Source: CAD feature listing. Evaluate the final solid. Frame: model axes, mm. Face numbers are marked on the shaded views. A direction names the side the tool comes from. Give positions to 0.01 mm unless a question says otherwise; leave off trailing zeros. Order: outer loops, then holes, each group sorted by start corner. A loop starts at its lowest first (then second) coordinate and runs counter-clockwise, first axis right, second up.
Autodesk Inventor part; units mm, degrees
ref_plane "YZ Plane" through (0, 0, 0) normal (1, 0, 0) x (0, 1, 0)
ref_plane "XZ Plane" through (0, 0, 0) normal (0, 1, 0) x (-1, 0, 0)
ref_plane "XY Plane" through (0, 0, 0) normal (0, 0, 1) x (1, 0, 0)
sketch "Sketch1" plane through (0, 0, 0) normal (0, 1, 0) x (-1, 0, 0)
  line L0 (-20.5, 52.5) -> (20.5, 52.5)
  line L1 (20.5, 52.5) -> (20.5, -52.5)
  line L2 (20.5, -52.5) -> (-20.5, -52.5)
  line L3 (-20.5, -52.5) -> (-20.5, 52.5)
  line L4 (-20.5, 52.5) -> (20.5, -52.5) construction
  line L5 (20.5, 52.5) -> (-20.5, -52.5) construction
  line L6 (-23.5, 55.5) -> (23.5, 55.5)
  line L7 (23.5, 55.5) -> (23.5, -55.5)
  line L8 (23.5, -55.5) -> (-23.5, -55.5)
  line L9 (-23.5, -55.5) -> (-23.5, 55.5)
  line L10 (-23.5, 55.5) -> (23.5, -55.5) construction
  line L11 (23.5, 55.5) -> (-23.5, -55.5) construction
  point P0 (0, 0)
  dimension "d0" = 41
  dimension "d1" = 105
  dimension "d4" = 47
  dimension "d5" = 111
extrude "Extrusion1" add sketch "Sketch1" along normal blind 3 contours L0 L1 L2 L3
sketch "Sketch3" plane through (0, 3, 0) normal (0, 1, 0) x (1, 0, 0)
  line L0 (23.5, -55.5) -> (-23.5, -55.5)
  line L1 (-23.5, -55.5) -> (-23.5, 55.5)
  line L2 (-23.5, 55.5) -> (23.5, 55.5)
  line L3 (23.5, 55.5) -> (23.5, -55.5)
  line L4 (23.5, -55.5) -> (-23.5, 55.5) construction
  line L5 (-23.5, -55.5) -> (23.5, 55.5) construction
  line L6 (20.5, 52.5) -> (-20.5, 52.5)
  line L7 (20.5, -52.5) -> (-20.5, -52.5)
  line L8 (-20.5, -52.5) -> (-20.5, 52.5)
  line L9 (-20.5, 52.5) -> (20.5, 52.5)
  line L10 (20.5, 52.5) -> (20.5, -52.5)
  line L11 (20.5, -52.5) -> (-20.5, 52.5) construction
  line L12 (-20.5, -52.5) -> (20.5, 52.5) construction
  point P0 (0, 0)
  dimension "d6" = 47
  dimension "d7" = 111
extrude "Extrusion3" add sketch "Sketch3" against normal blind 65
sketch "Sketch4" plane through (23.5, 3, -55.5) normal (0, 0, -1) x (-1, 0, 0)
  line L0 (0, 0) -> (23.5, 0) construction
  line L1 (23.5, 0) -> (23.5, -48) construction
  line L2 (23.5, -48) -> (14.75, -48) construction
  line L3 (23.5, -48) -> (32.25, -48) construction
  circle A0 centre (14.75, -48) radius 2
  circle A1 centre (32.25, -48) radius 2
  point P0 (23.5, -3)
  dimension "d12" = 23.5
  dimension "d13" = 48
  dimension "d14" = 8.75
  dimension "d15" = 8.75
  dimension "d16" = 4
  dimension "d17" = 4
extrude "Extrusion4" cut sketch "Sketch4" against normal blind 3
sketch "Sketch5" plane through (-23.5, 3, 55.5) normal (0, 0, 1) x (1, 0, 0)
  line L0 (47, 0) -> (47, -65) construction
  line L1 (47, 0) -> (23.5, 0) construction
  line L2 (0, 0) -> (47, 0) construction
  line L3 (23.5, 0) -> (23.5, -48) construction
  line L4 (23.5, 0) -> (71.5, 0) construction
  circle A0 centre (32.25, -48) radius 2
  line L5 (23.5, -48) -> (32.25, -48) construction
  circle A1 centre (14.75, -48) radius 2
  line L6 (23.5, -48) -> (14.75, -48) construction
  circle A2 centre (32.25, -48) radius 2 construction
  circle A3 centre (14.75, -48) radius 2 construction
  point P0 (23.5, -3)
  dimension "d20" = 23.5
  dimension "d21" = 48
  dimension "d22" = 90
extrude "Extrusion5" cut sketch "Sketch5" against normal blind 3
sketch "Sketch6" plane through (23.5, 3, 55.5) normal (1, 0, 0) x (0, 0, -1)
  line L0 (111, 0) -> (111, -65) construction
  line L1 (111, 0) -> (55.5, 0) construction
  line L2 (111, 0) -> (0, 0) construction
  line L3 (55.5, 0) -> (51.5, 0) construction
  line L4 (51.5, 0) -> (59.5, 0)
  line L5 (59.5, 0) -> (59.5, -8)
  line L6 (59.5, -8) -> (51.5, -8)
  line L7 (51.5, -8) -> (51.5, 0)
  line L8 (51.5, 0) -> (47.5, 0)
  line L9 (47.5, 0) -> (45.5, 0)
  line L10 (45.5, 0) -> (45.5, -8)
  line L11 (45.5, -8) -> (47.5, -8)
  line L12 (47.5, -8) -> (47.5, 0)
  line L13 (59.5, 0) -> (63.5, 0)
  line L14 (63.5, 0) -> (65.5, 0)
  line L15 (65.5, 0) -> (65.5, -8)
  line L16 (65.5, -8) -> (63.5, -8)
  line L17 (63.5, -8) -> (63.5, 0)
  point P0 (55.5, -3)
  dimension "d25" = 55.5
  dimension "d26" = 4
  dimension "d27" = 8
  dimension "d28" = 8
  dimension "d29" = 4
  dimension "d30" = 2
  dimension "d31" = 4
  dimension "d32" = 2
  dimension "d33" = 8
extrude "Extrusion6" cut sketch "Sketch6" against normal blind 3
sketch "Sketch7" plane through (20.5, 3, 55.5) normal (1, 0, 0) x (0, 0, -1)
  point P0 (55.5, -3)
sketch "Sketch8" plane through (20.5, 3, 55.5) normal (1, 0, 0) x (0, 0, -1)
  line L0 (65.5, 0) -> (65.5, -3)
  line L1 (63.5, -3) -> (59.5, -3)
  line L2 (65.5, 0) -> (63.5, 0)
  line L3 (63.5, 0) -> (63.5, -3)
  line L4 (63.5, -3) -> (65.5, -3)
  line L5 (65.5, -3) -> (65.5, 0)
  line L6 (51.5, 0) -> (59.5, 0)
  line L7 (51.5, -3) -> (51.5, 0)
  line L8 (59.5, 0) -> (51.5, 0)
  line L9 (51.5, 0) -> (51.5, -3)
  line L10 (51.5, -3) -> (59.5, -3)
  line L11 (59.5, -3) -> (59.5, 0)
  line L12 (51.5, 0) -> (47.5, 0)
  line L13 (45.5, -8) -> (45.5, 0)
  line L14 (47.5, 0) -> (45.5, 0)
  line L15 (45.5, 0) -> (45.5, -3)
  line L16 (45.5, -3) -> (47.5, -3)
  line L17 (47.5, -3) -> (47.5, 0)
  point P0 (55.5, -3)
extrude "Extrusion7" add sketch "Sketch8" along normal blind 3
sketch "Sketch9" plane through (23.5, 3, 55.5) normal (1, 0, 0) x (0, 0, -1)
  line L0 (59.5, -8) -> (51.5, -8)
  circle A0 centre (55.5, -8) radius 4
  point P0 (55.5, -3)
  dimension "d38" = 8
extrude "Extrusion8" cut sketch "Sketch9" against normal blind 3
sketch "Sketch10" plane through (0, 3, 0) normal (0, 1, 0) x (1, 0, 0)
  line L0 (-23.5, 55.5) -> (23.5, 55.5)
  line L1 (0, 55.5) -> (0, 40.5) construction
  line L2 (0, 40.5) -> (0, 35.5) construction
  line L3 (0, 35.5) -> (0, 30.5) construction
  line L4 (0, 30.5) -> (0, 25.5) construction
  line L5 (0, 25.5) -> (0, 20.5) construction
  line L6 (0, 20.5) -> (0, 15.5) construction
  line L7 (0, 15.5) -> (0, 10.5) construction
  line L8 (0, 10.5) -> (0, 5.5) construction
  line L9 (0, 5.5) -> (0, 0.5) construction
  line L10 (-15, 1.5) -> (15, 1.5)
  line L11 (15, 1.5) -> (15, -1.5)
  line L12 (15, -1.5) -> (-15, -1.5)
  line L13 (-15, -1.5) -> (-15, 1.5)
  line L14 (-15, 1.5) -> (15, -1.5) construction
  line L15 (15, 1.5) -> (-15, -1.5) construction
  line L16 (-15, 7) -> (15, 7)
  line L17 (15, 7) -> (15, 4)
  line L18 (15, 4) -> (-15, 4)
  line L19 (-15, 4) -> (-15, 7)
  line L20 (-15, 7) -> (15, 4) construction
  line L21 (15, 7) -> (-15, 4) construction
  line L22 (-15, 12) -> (15, 12)
  line L23 (15, 12) -> (15, 9)
  line L24 (15, 9) -> (-15, 9)
  line L25 (-15, 9) -> (-15, 12)
  line L26 (-15, 12) -> (15, 9) construction
  line L27 (15, 12) -> (-15, 9) construction
  line L28 (-15, 17) -> (15, 17)
  line L29 (15, 17) -> (15, 14)
  line L30 (15, 14) -> (-15, 14)
  line L31 (-15, 14) -> (-15, 17)
  line L32 (-15, 17) -> (15, 14) construction
  line L33 (15, 17) -> (-15, 14) construction
  line L34 (-15, 22) -> (15, 22)
  line L35 (15, 22) -> (15, 19)
  line L36 (15, 19) -> (-15, 19)
  line L37 (-15, 19) -> (-15, 22)
  line L38 (-15, 22) -> (15, 19) construction
  line L39 (15, 22) -> (-15, 19) construction
  line L40 (-15, 27) -> (15, 27)
  line L41 (15, 27) -> (15, 24)
  line L42 (15, 24) -> (-15, 24)
  line L43 (-15, 24) -> (-15, 27)
  line L44 (-15, 27) -> (15, 24) construction
  line L45 (15, 27) -> (-15, 24) construction
  line L46 (-15, 32) -> (15, 32)
  line L47 (15, 32) -> (15, 29)
  line L48 (15, 29) -> (-15, 29)
  line L49 (-15, 29) -> (-15, 32)
  line L50 (-15, 32) -> (15, 29) construction
  line L51 (15, 32) -> (-15, 29) construction
  line L52 (-15, 37) -> (15, 37)
  line L53 (15, 37) -> (15, 34)
  line L54 (15, 34) -> (-15, 34)
  line L55 (-15, 34) -> (-15, 37)
  line L56 (-15, 37) -> (15, 34) construction
  line L57 (15, 37) -> (-15, 34) construction
  line L58 (-15, 42) -> (15, 42)
  line L59 (15, 42) -> (15, 39)
  line L60 (15, 39) -> (-15, 39)
  line L61 (-15, 39) -> (-15, 42)
  line L62 (-15, 42) -> (15, 39) construction
  line L63 (15, 42) -> (-15, 39) construction
  point P0 (0, 0)
  dimension "d41" = 15
  dimension "d42" = 5
  dimension "d43" = 5
  dimension "d44" = 5
  dimension "d45" = 5
  dimension "d46" = 5
  dimension "d47" = 5
  dimension "d48" = 5
  dimension "d49" = 5
  dimension "d50" = 30
  dimension "d51" = 3
  dimension "d52" = 30
  dimension "d53" = 3
  dimension "d54" = 30
  dimension "d55" = 3
  dimension "d56" = 30
  dimension "d57" = 3
  dimension "d58" = 30
  dimension "d59" = 3
  dimension "d60" = 30
  dimension "d61" = 3
  dimension "d62" = 30
  dimension "d63" = 3
  dimension "d64" = 30
  dimension "d65" = 3
  dimension "d66" = 30
  dimension "d67" = 3
extrude "Extrusion9" cut sketch "Sketch10" against normal blind 3
properties part number "netzteil_case"
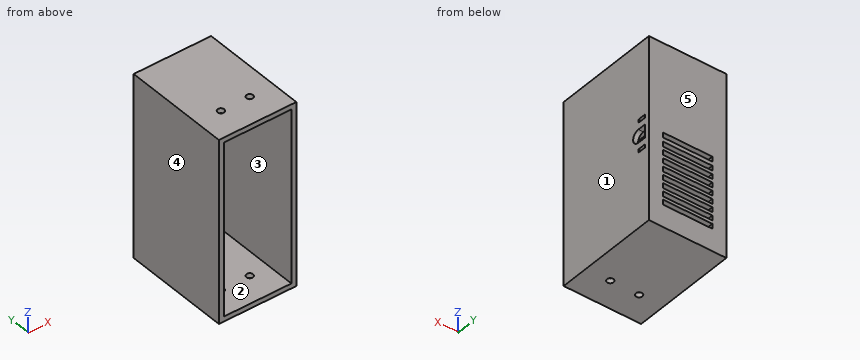
(1) Section A-A, the plane y = -45. Return loops of the section in (x, z), plus the area to 3 significant figures.
(2) Pin query (flat end, axial travel): pin 1 Ø4 at (x, z) = (15, 38) entering from -Y. Return the tip coordinate at first contact, or that it passes through.
(3) Section D-D, the plane x = 0. Count the separate pieces of the cut face and the enclosed holes in it, plus the area to 3 significant figures.
(4) Draft query along X for the marked faces 3, 4 and 5. Return one class per face: +X half, -X half, draft (parallel to the pull), parting line (faces both ways), or undercut.
(5) Section C-C, the plane y = -57. Return loops of the section in (x, z), plus the area to 3 significant figures.
(6) Section B-B, the plane z = 42. Return loops of the section in (x, y).
(7) Access query for the marked faces 1 and 2. Directions: +Z, -Z, +X, -X, +Y, -Y. A direction counts if a zero-diameter tool reaches every point of the face in a straight line with its end or side. Return the directions, or none.
(8) Line query: line 1 along Z through (x, y) = (9.5, -52.5); line 2 along X through (y, z) = (-52, 37.5); line 3 along Y through (x, z) = (-8.75, -53.6). Output: solid intervals per line, ascending.
Checks:
1. outline: (-23.5, -55.5) - (-10.75, -55.5) - (-10.75, -52.5) - (-20.5, -52.5) - (-20.5, 52.5) - (-10.75, 52.5) - (-10.75, 55.5) - (-23.5, 55.5) - close; (-6.75, -55.5) - (6.75, -55.5) - (6.75, -52.5) - (-6.75, -52.5) - close; (-6.75, 52.5) - (6.75, 52.5) - (6.75, 55.5) - (-6.75, 55.5) - close; (10.75, -55.5) - (23.5, -55.5) - (23.5, 55.5) - (10.75, 55.5) - (10.75, 52.5) - (20.5, 52.5) - (20.5, -52.5) - (10.75, -52.5) - close
1. area: 864 mm2
2. pin 1: stops at y = 0
3. separate pieces: 10
3. enclosed holes: 0
3. area: 624 mm2
4. face 3: undercut
4. face 4: -X half
4. face 5: draft
5. outline: (-23.5, -55.5) - (23.5, -55.5) - (23.5, 55.5) - (-23.5, 55.5) - close; hole (-20.5, -52.5) - (20.5, -52.5) - (20.5, 52.5) - (-20.5, 52.5) - close
5. area: 912 mm2
6. outline: (-23.5, -62) - (-20.5, -62) - (-20.5, 0) - (20.5, 0) - (20.5, -62) - (23.5, -62) - (23.5, 3) - (-23.5, 3) - close
7. face 1: +Z, -Z, +X, +Y, -Y
7. face 2: -Y
8. line 1: z = -55.5 to -52.5, 52.5 to 55.5
8. line 2: x = -23.5 to -20.5, 20.5 to 23.5
8. line 3: y = -62 to -47, -43 to 3
